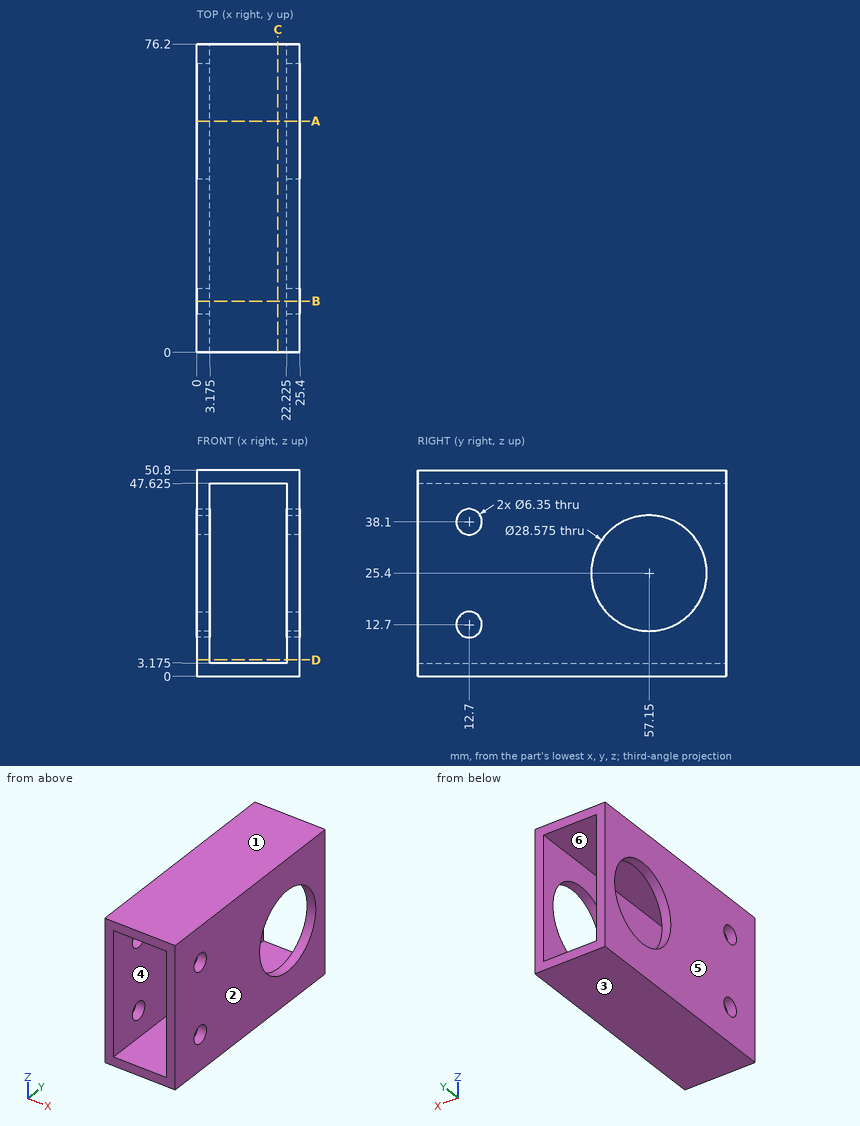
Study the drawing (mm; zero at the part's minimum x, y, z) and answer. A direction names the side the tool comes from. Give positions to 0.01 mm unless a question says otherwise; leave off trailing zeros. Order: outer loops, then holes, each group sorted by start corner. A loop starts at its lowest first (then second) coordinate and runs counter-clockwise, first axis right, second up.
1. Section B-B, the plane y = 12.7 is taken. Determine the outline of the cut face in (x, z) (3 decimals), and give its area (3 significant figures).
Result sheet:
outline: (0, 0) - (25.4, 0) - (25.4, 9.525) - (22.225, 9.525) - (22.225, 3.175) - (3.175, 3.175) - (3.175, 9.525) - (0, 9.525) - close; (0, 15.875) - (3.175, 15.875) - (3.175, 34.925) - (0, 34.925) - close; (0, 41.275) - (3.175, 41.275) - (3.175, 47.625) - (22.225, 47.625) - (22.225, 41.275) - (25.4, 41.275) - (25.4, 50.8) - (0, 50.8) - close; (22.225, 15.875) - (25.4, 15.875) - (25.4, 34.925) - (22.225, 34.925) - close
area: 363 mm2
2. Each of these flat-tipped pins is pushed along its axis until it touches: P1, Ø5, axis at x = 6, z = 7.5, coming from the +Y side; P2, Ø2, axis at y = 40, z = 7.5, coming from the -X side. Where does it stop, or does it pass through?
Result sheet:
P1: passes through
P2: stops at x = 0
3. Straight lines are drawn through the part: L1, parallel to Y at x = 23.1, z = 25.4; L2, parallel to Z at x = 10.25, y = 58.5 (3 decimals); L3, parallel to Z at x = 22.5, y = 57. For each, find the intervals that lie inside material, in ascending order.
Result sheet:
L1: y = 0 to 42.86, 71.44 to 76.2
L2: z = 0 to 3.175, 47.625 to 50.8
L3: z = 0 to 11.11, 39.69 to 50.8
4. For the marked faces 5 and 6, determine the directions among +Z, -Z, +X, -X, +Y, -Y from which every point of the face is accessible in a straight line to the end or side of a thin tool.
Result sheet:
face 5: +Z, -Z, -X, +Y, -Y
face 6: +Y, -Y
5. The mould has two halves that part along Z. Classify the marked faces 1, 2, 3 and 4: released by +Z, released by -Z, zero draft, split by the parting line, or undercut.
Result sheet:
face 1: released by +Z
face 2: zero draft
face 3: released by -Z
face 4: undercut
6. Section A-A, the plane y = 57.15 is taken. Determine the outline of the cut face in (x, z) (1 decimal).
Result sheet:
outline: (0, 0) - (25.4, 0) - (25.4, 11.1) - (22.2, 11.1) - (22.2, 3.2) - (3.2, 3.2) - (3.2, 11.1) - (0, 11.1) - close; (0, 39.7) - (3.2, 39.7) - (3.2, 47.6) - (22.2, 47.6) - (22.2, 39.7) - (25.4, 39.7) - (25.4, 50.8) - (0, 50.8) - close
7. Section D-D, the plane z = 4 is taken. Determine the outline of the cut face in (x, y) (3 decimals), and give its area (3 significant figures).
Result sheet:
outline: (0, 0) - (3.175, 0) - (3.175, 76.2) - (0, 76.2) - close; (22.225, 0) - (25.4, 0) - (25.4, 76.2) - (22.225, 76.2) - close
area: 484 mm2
8. Section C-C, the plane x = 20 is taken. Determine the outline of the cut face in (y, z) (3 decimals).
Result sheet:
outline: (0, 0) - (76.2, 0) - (76.2, 3.175) - (0, 3.175) - close; (0, 47.625) - (76.2, 47.625) - (76.2, 50.8) - (0, 50.8) - close
